from build123d import *

# Parameters (mm, degrees)
BOSS_EXTRUDE1_DEPTH = 6.096
SKETCH3_R           = 12.5
CUT_EXTRUDE1_DEPTH  = 44.45
SKETCH4_R           = 12.5
CUT_EXTRUDE2_DEPTH  = 6.096


with BuildPart() as part:
    # Sketch1 → Boss-Extrude1 (new body)
    with BuildSketch(Plane(origin=(0, 0, 0), x_dir=(1, 0, 0), z_dir=(0, 1, 0))):
        Polygon((-63.779220614, -177.8), (-190.779220614, 0), (-63.779220614, 177.8), (63.779220614, 177.8), (63.779220614, -177.8), align=None)
    extrude(amount=BOSS_EXTRUDE1_DEPTH)

    # Sketch3 → Cut-Extrude1 (cut)
    with BuildSketch(Plane(origin=(0, 6.096, 0), x_dir=(1, 0, 0), z_dir=(0, 1, 0))):
        with Locations(Location((-143.5, 0, 0), (0, 0, 270))):
            Circle(SKETCH3_R)
        with Locations(Location((16.5, 0, 0), (0, 0, 270))):
            Circle(SKETCH3_R)
    extrude(amount=-CUT_EXTRUDE1_DEPTH, mode=Mode.SUBTRACT)

    # Sketch4 → Cut-Extrude2 (cut)
    with BuildSketch(Plane.XZ):
        with Locations(Location((12.979220614, 127, 0), (0, 0, 270))):
            Circle(SKETCH4_R)
        with Locations(Location((12.979220614, -127, 0), (0, 0, 90))):
            Circle(SKETCH4_R)
    extrude(amount=-CUT_EXTRUDE2_DEPTH, mode=Mode.SUBTRACT)


solid = part.part
The model under review builds one solid part; all positions refer to its coordinate system, in mm. Round coordinates to 2 decimals unless told otherwise and drop trailing zeros. Loops run counter-clockwise (first coordinate to the right, second up) from the corner with the lowest first, then second, coordinate; pieces in that order, holes last. Notation, with made-up numbers: (22.5, 2.5) -> (42.5, 2.5) arc R28 ccw to (42.5, 34.5) -> close; hole circle Ø9 at (-34.5, 63.5). An arc over 180 degrees is marked (long way). Return JSON: item names as keys, results as strings.
(1) Add section A-A on z = 7. Write out the cut boundary in (x, y).
Solved:
{"outline": "(-185.78, 0) -> (-153.86, 0) -> (-153.86, 6.1) -> (-185.78, 6.1) -> close; (-133.14, 0) -> (6.14, 0) -> (6.14, 6.1) -> (-133.14, 6.1) -> close; (26.86, 0) -> (63.78, 0) -> (63.78, 6.1) -> (26.86, 6.1) -> close"}
(2) The part is to be moulded in two halves that separate along Z. For faces 1 (the flat face through (-126.39, 3.005, 90.145)), 2 (the cylindrical face through (5.41, 3.09, 5.77)), 3 (the flat face through (-33, 6.096, -2)), say which applies: released by +Z, released by -Z, zero draft, split by the parting line, or undercut.
Solved:
{"face 1": "released by +Z", "face 2": "undercut", "face 3": "zero draft"}
(3) Add section D-D on x = -143.5. Write out the cut boundary in (y, z), plus the area to 3 significant figures.
Solved:
{"outline": "(0, -66.19) -> (6.1, -66.19) -> (6.1, -12.5) -> (0, -12.5) -> close; (0, 12.5) -> (6.1, 12.5) -> (6.1, 66.19) -> (0, 66.19) -> close", "area": "655 mm2"}
(4) Add section B-B on y = 2. Write out the cut boundary in (x, z), plus the area to 3 significant figures.
Solved:
{"outline": "(-190.78, 0) -> (-63.78, -177.8) -> (63.78, -177.8) -> (63.78, 177.8) -> (-63.78, 177.8) -> close; hole circle Ø25 at (-143.5, 0); hole circle Ø25 at (12.98, -127); hole circle Ø25 at (12.98, 127); hole circle Ø25 at (16.5, 0)", "area": "66,000 mm2"}
(5) Add section C-C on x = 16.5. Write out the cut boundary in (y, z).
Solved:
{"outline": "(0, -177.8) -> (6.1, -177.8) -> (6.1, -138.99) -> (0, -138.99) -> close; (0, -115.01) -> (6.1, -115.01) -> (6.1, -12.5) -> (0, -12.5) -> close; (0, 12.5) -> (6.1, 12.5) -> (6.1, 115.01) -> (0, 115.01) -> close; (0, 138.99) -> (6.1, 138.99) -> (6.1, 177.8) -> (0, 177.8) -> close"}
(6) For line 1 (X direction, y = 2, z = 0); line 2 (Z direction, x = 22, y = 2.25); line 3 (X direction, y = 2, z = 5.5), list the stretches that pass through material, from the lowest coordinate up.
Solved:
{"line 1": "-190.78 to -156, -131 to 4, 29 to 63.78", "line 2": "-177.8 to -135.65, -118.35 to -11.22, 11.22 to 118.35, 135.65 to 177.8", "line 3": "-186.85 to -154.72, -132.28 to 5.28, 27.72 to 63.78"}
